The model under review builds one solid part; all positions refer to its coordinate system, in mm. Face numbers are marked on the shaded views. A direction names the side the tool comes from. Round coordinates to 2 decimals unless told otherwise and drop trailing zeros. Order: outer loops, then holes, each group sorted by start corner. A loop starts at its lowest first (then second) coordinate and runs counter-clockwise, first axis right, second up.
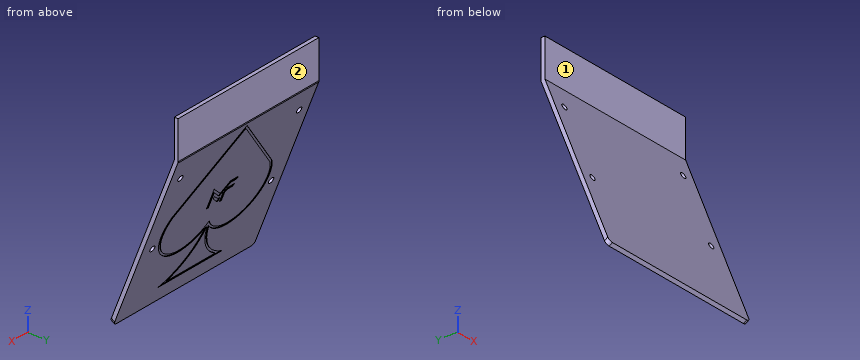
```python
from build123d import *

# Parameters (mm, degrees)
RESSALTO_EXTRUS_O1_DEPTH = 87.78
ESBO_O2_R                = 1.55
CORTE_EXTRUS_O1_DEPTH    = 2.000797456
FILETE1_R                = 2
FILETE2_R                = 2
CORTE_EXTRUS_O2_DEPTH    = 0.3
CORTE_EXTRUS_O3_DEPTH    = 0.3


with BuildPart() as part:
    # Esboço1 → Ressalto-extrusão1 (new body)
    with BuildSketch(Plane(origin=(0, 0, 0), x_dir=(0, 0, -1), z_dir=(1, 0, 0))):
        Polygon((0, 2), (19.99, 2), (106.12, -31.745348352), (105.11, -33.498517173), (19.61, 0), (0, 0), align=None)
    extrude(amount=RESSALTO_EXTRUS_O1_DEPTH)

    # Esboço2 → Corte-extrusão1 (cut)
    with BuildSketch(Plane(origin=(0, 8.523589674, -3.33950427), x_dir=(1, 0, 0), z_dir=(0, 0.9310875040982999, -0.36479591515256676))):
        with Locations(Location((80.80000159, 30.587577749, 0), (0, 0, 270))):
            Circle(ESBO_O2_R)
        with Locations(Location((6.80000159, 30.587577749, 0), (0, 0, 270))):
            Circle(ESBO_O2_R)
        with Locations(Location((80.80000159, 70.587577749, 0), (0, 0, 270))):
            Circle(ESBO_O2_R)
        with Locations(Location((6.80000159, 70.587577749, 0), (0, 0, 270))):
            Circle(ESBO_O2_R)
    extrude(amount=-CORTE_EXTRUS_O1_DEPTH, mode=Mode.SUBTRACT)

    # Filete1
    filete1_edges = [part.edges().sort_by_distance(p)[0] for p in [
        (87.78, -32.621932763, -105.615),
        (0, -32.621932763, -105.615),
    ]]
    fillet(filete1_edges, radius=FILETE1_R)

    # Filete2
    filete2_edges = [part.edges().sort_by_distance(p)[0] for p in [
        (43.89, 2, -19.99),
    ]]
    fillet(filete2_edges, radius=FILETE2_R)

    # Esboço5 → Corte-extrusão2 (cut)
    with BuildSketch(Plane(origin=(0, 8.523589674, -3.33950427), x_dir=(1, 0, 0), z_dir=(0, 0.9310875040982999, -0.36479591515256676))):
        with BuildLine():
            ThreePointArc((42.554958064, 77.750017871), (36.485484967, 92.178478749), (23.83842585, 101.401866557))
            Line((23.83842585, 101.401866557), (63.94157415, 101.401866557))
            ThreePointArc((63.94157415, 101.401866557), (51.294515033, 92.178478749), (45.225041936, 77.750017871))
            ThreePointArc((45.225041936, 77.750017871), (70.022049562, 80.317662999), (75.100625445, 55.910851333))
            Line((75.100625445, 55.910851333), (43.890007976, 19.871588801))
            Line((43.890007976, 19.871588801), (12.680587753, 55.908777517))
            ThreePointArc((12.680587753, 55.908777517), (17.756980644, 80.316954028), (42.554958064, 77.750017871))
        make_face()
        with BuildLine():
            Line((59.045444566, 100.301866557), (28.734555434, 100.301866557))
            ThreePointArc((28.734555434, 100.301866557), (38.853768409, 90.783324538), (43.663553306, 77.750017871))
            Line((43.663553306, 77.750017871), (44.116446694, 77.750017871))
            ThreePointArc((44.116446694, 77.750017871), (48.926231591, 90.783324538), (59.045444566, 100.301866557))
        make_face(mode=Mode.SUBTRACT)
        with BuildLine():
            ThreePointArc((43.89, 74.051866557), (19.984051861, 80.457020374), (13.579692383, 56.550859421))
            Line((13.579692383, 56.550859421), (43.89, 21.551866557))
            Line((43.89, 21.551866557), (74.201470581, 56.552873732))
            ThreePointArc((74.201470581, 56.552873732), (67.794940984, 80.457601856), (43.89, 74.051866557))
        make_face(mode=Mode.SUBTRACT)
    extrude(amount=-CORTE_EXTRUS_O2_DEPTH, mode=Mode.SUBTRACT)

    # Logo_MF → Corte-extrusão3 (cut)
    with BuildSketch(Plane(origin=(0, 8.523589674, -3.33950427), x_dir=(1, 0, 0), z_dir=(0, 0.9310875040982999, -0.36479591515256676))):
        Polygon((49.962573353, 64.155016633), (48.8289818, 64.155016633), (48.8289818, 55.535121255), (43.89, 60.021613531), (38.906920465, 54.778752605), (35.388063353, 54.778752605), (34.260081833, 53.537007416), (39.45058041, 53.537007416), (43.888190467, 58.422176933), (49.962573353, 52.904304422), align=None)
        Polygon((47.520333519, 58.27431755), (47.520333519, 59.844814175), (43.63988582, 63.369750961), (42.9589818, 62.620173706), (42.9589818, 60.900053981), (43.641004718, 61.650862981), align=None)
        Polygon((41.8589818, 64.155016633), (41.8589818, 59.312995139), (39.859003533, 57.208752605), (35.175514937, 57.208752605), (36.327896381, 58.421210806), (39.450099751, 58.421210806), (40.643954402, 59.677304324), (40.643954402, 64.155016633), align=None)
    extrude(amount=-CORTE_EXTRUS_O3_DEPTH, mode=Mode.SUBTRACT)


solid = part.part
```
(1) For the marked faces 1 and 2, list the 3-axis set-ups (+Z, -Z, +X, -X, +Y, -Y) from which the entire face can be reached by the end or side of a thin tool; tool diameter is ignored.
Data:
face 1: +Z, +X, -X, -Y
face 2: +Z, -Z, +X, -X, +Y
(2) Consider section C-C (x = 25). Write out the cut boundary in (y, z).
Data:
outline: (-33.5, -105.11) - (-31.75, -106.12) - (-28.47, -97.75) - (-28.75, -97.64) - (-28.58, -97.21) - (-28.3, -97.32) - (-21.95, -81.11) - (-22.22, -81) - (-21.81, -79.95) - (-21.54, -80.06) - (-7.3, -43.72) - (-7.57, -43.61) - (-6.96, -42.04) - (-6.68, -42.15) - (1.86, -20.34) arc R2 ccw to (2, -19.61) - (2, 0) - (0, 0) - (0, -19.61) - close
(3) Insertion check: pin 1 (15.5 mm diameter, centred on x = 53, z = -8.5, fed in from -Y); pin 2 (1.5 mm diameter, centred on x = 77.5, z = -50.5, fed in from -Y). Each pin has a flat end and moves straight along its axis. Give the tip position at first contact, or say it passes through.
Data:
pin 1: stops at y = 0
pin 2: stops at y = -12.4
(4) To check wall thickness, follow probe 1 along Y at (x, z) = (77, -18.5); probe 2 along Y at (x, z) = (36.5, -101.5). State the ranges of each line that lie inside material, in increasing order.
Data:
probe 1: y = 0 to 2
probe 2: y = -32.08 to -29.94
(5) Consider section A-A (z = -38). Write out the cut boundary in (x, y).
Data:
outline: (0, -7.21) - (87.78, -7.21) - (87.78, -5.06) - (58.92, -5.06) - (59.02, -5.38) - (57.57, -5.38) - (57.46, -5.06) - (30.32, -5.06) - (30.21, -5.38) - (28.76, -5.38) - (28.86, -5.06) - (0, -5.06) - close
(6) Consider section B-B (x = 66). Write out the cut boundary in (y, z).
Data:
outline: (-33.5, -105.11) - (-31.75, -106.12) - (-21.59, -80.2) - (-21.87, -80.09) - (-21.44, -78.98) - (-21.16, -79.09) - (-8.65, -47.18) - (-8.93, -47.07) - (-8.32, -45.5) - (-8.04, -45.61) - (1.86, -20.34) arc R2 ccw to (2, -19.61) - (2, 0) - (0, 0) - (0, -19.61) - close
